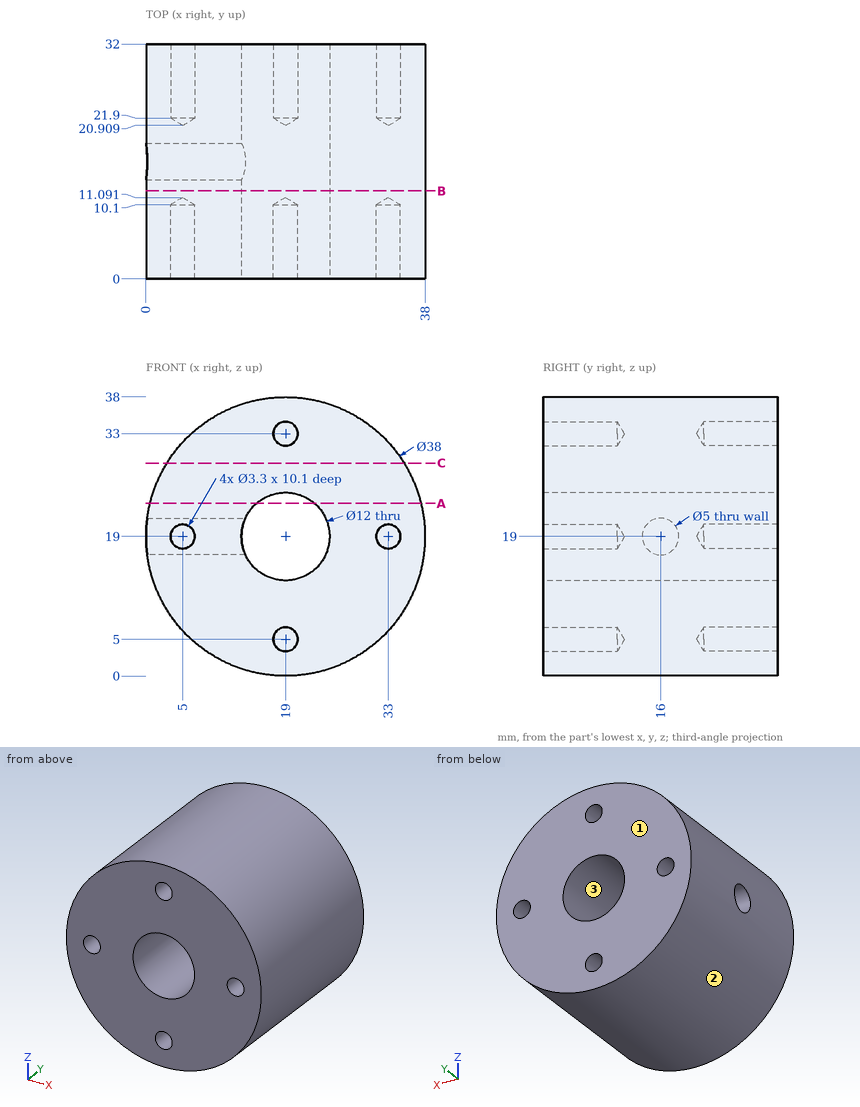
Check sheet for the drawn part. Datum: minimum x, y, z corner. Units: mm. Round coordinates to 2 decimals unless told otherwise and drop trailing zeros. Order: outer loops, then holes, each group sorted by start corner. A loop starts at its lowest first (then second) coordinate and runs counter-clockwise, first axis right, second up. Notation, with made-up numbers: (8.5, 9.25) - (26.5, 9.25) arc R12 ccw to (26.5, 25.25) - close; hole circle Ø10 at (39, 50.5). An arc over 180 degrees is marked (long way). Use a Markdown table: item, result. Add a question column.
(1) Sectioned sample at C-C, the plane z = 29. Enter the section's corners in (x, y) (1 decimal), and give its area (3 significant figures).
(2) Material ranges on line 1 along X through (y, z) = (10, 15) (1 decimal); line 2 along X through (y, z) = (9.5, 6) (1 decimal); line 3 along Z through (x, y) = (2, 27) (1 decimal), recorded low to high. Write a range as [from, to].
(3) Sectioned sample at A-A, the plane z = 23.5. Enter the section's corners in (x, y).
(4) Sectioned sample at B-B, the plane y = 12. Enter the section's corners in (x, z), and give its area (3 significant figures).
(5) Release check for a two-part mould opening along Z. For the marked faces 1, 2 and 3 record: pulls with the +Z half, pulls with the -Z half, needs draft (parallel to the pull), parting line crosses it, or undercut.
(6) Depth check by flat-ended pin: pin 1 (10 mm diameter, centred on y = 4.5, z = 31.5, fed in from +X); pin 2 (6 mm diameter, centred on y = 16, z = 19, fed in from +X); pin 3 (8 mm diameter, centred on y = 11, z = 27.5, fed in from -X). Enter the tip coordinate at first touch or a pass-through.
Answers below:
| question | item | result |
|---|---|---|
| 1 | outline | (2.8, 0) - (35.2, 0) - (35.2, 32) - (2.8, 32) - close |
| 1 | area | 1,030 mm² |
| 2 | line 1 | [0.4, 14.5], [23.5, 37.6] |
| 2 | line 2 | [5.1, 17.7], [20.3, 32.9] |
| 2 | line 3 | [10.5, 27.5] |
| 3 | outline | (0.54, 0) - (15.03, 0) - (15.03, 32) - (0.54, 32) - close; (22.97, 0) - (37.46, 0) - (37.46, 32) - (22.97, 32) - close |
| 4 | outline | circle Ø38 at (19, 19); hole circle Ø12 at (19, 19) |
| 4 | area | 1,020 mm² |
| 5 | face 1 | needs draft |
| 5 | face 2 | parting line crosses it |
| 5 | face 3 | undercut |
| 6 | pin 1 | x = 36.46 |
| 6 | pin 2 | x = 38 |
| 6 | pin 3 | x = 0.54 |
